Could you check a few things on this model? Use its own coordinates, in mm. A direction names the side the tool comes from. Give positions to 0.01 mm unless a question says otherwise; leave off trailing zeros. Loops run counter-clockwise (first coordinate to the right, second up) from the corner with the lowest first, then second, coordinate; pieces in that order, holes last. Notation, with made-up numbers: (70, 11.25) - (79, 11.25) arc R36 ccw to (79, 45.25) - close; hole circle Ø1 at (26, 47.25). An arc over 180 degrees is marked (long way). Write each question's results on one line, items separated by ' | '. Start each with the question number.
(1) Suppose I cut it at B-B (y = 20). Please give me the cut outline in (x, z).
(2) If we mould it in two halves opening along X, with no side actions, what happens to faces 1 (the face through (-17.7, 43.22, 87.97)), 2 (the face through (52, 43, 117.475)), 3 (the face through (-25.4, 43, 27))? For each: released by +X, released by -X, zero draft, split by the parting line, or undercut.
(3) On a 3-axis mill with a long thin cutter (end or side, diameter ignored), from which of +Z, -Z, +X, -X, +Y, -Y can I reach the whole of each face in a straight line? I mean faces 4 (the face through (0, 20, 3)), 5 (the face through (101.6, 20, 3)), 6 (the face through (50, 20, 6.35)), 7 (the face through (3.175, 43, -39)). Say none if no direction works.
(4) Suppose I cut it at D-D (x = 39). Please give me the cut outline in (y, z) (3 decimals).
(5) Suppose I cut it at C-C (y = 42). Please give me the cut outline in (x, z) (3 decimals), and give its area (3 significant figures).
(6) For pin 1 (20 mm diameter, centred on x = 56.5, y = 18.5, fed in from -Z); pin 2 (2.5 mm diameter, centred on x = 119.2, z = 85.725, fed in from +Y); pin 3 (7 mm diameter, centred on x = 45.5, y = 42, fed in from -Z) (3 decimals); pin 4 (14.5 mm diameter, centred on x = 12.7, y = 20, fed in from +Z), each with a flat end and sliding along its axis, tell me the tip position at first contact or that it passes through.
(7) Suppose I cut it at A-A (x = 88.9). Please give me the cut outline in (y, z) (3 decimals).
(8) I need wall thicknesses on line 1 (X direction, y = 20, z = 1.5); line 2 (Z direction, x = -17.6, y = 44.25) (3 decimals); line 3 (Y direction, x = 64, z = 12.5). Which ranges of each line are inside material? Lowest first, please.
Autodesk Inventor part; units mm, degrees
ref_plane "YZ Plane" through (0, 0, 0) normal (1, 0, 0) x (0, 1, 0)
ref_plane "XZ Plane" through (0, 0, 0) normal (0, 1, 0) x (-1, 0, 0)
ref_plane "XY Plane" through (0, 0, 0) normal (0, 0, 1) x (1, 0, 0)
sketch "Sketch1" plane through (0, 0, 0) normal (0, 0, 1) x (1, 0, 0)
  line L0 (0, 0) -> (101.6, 0)
  line L1 (101.6, 0) -> (101.6, 40)
  line L2 (101.6, 40) -> (0, 40)
  line L3 (0, 40) -> (0, 0)
  dimension "d0" = 101.6
  dimension "d1" = 40
extrude "Mounting Plate" add sketch "Sketch1" along normal blind 6.35
sketch "Sketch2" plane through (0, 40, 0) normal (0, 1, 0) x (1, 0, 0)
  line L0 (0, -6.35) -> (101.6, -6.35)
  line L1 (101.6, 0) -> (101.6, -6.35)
  line L2 (101.6, 0) -> (0, 0)
  line L3 (0, 0) -> (0, -6.35)
  line L4 (-25.4, 66.675) -> (127, 66.675)
  line L5 (127, 66.675) -> (127, -117.475)
  line L6 (127, -117.475) -> (-25.4, -117.475)
  line L7 (-25.4, -117.475) -> (-25.4, 66.675)
  line L8 (3.175, 66.675) -> (98.425, 66.675)
  line L9 (98.425, 66.675) -> (98.425, 12.7)
  line L10 (95.25, 9.525) -> (6.35, 9.525)
  line L11 (3.175, 12.7) -> (3.175, 66.675)
  arc A0 (3.175, 12.7) -> (6.35, 9.525) centre (6.35, 12.7) ccw
  arc A1 (95.25, 9.525) -> (98.425, 12.7) centre (95.25, 12.7) ccw
  point P0 (98.425, 9.525)
  point P1 (3.175, 9.525)
  point P2 (50.8, 66.675)
  point P3 (50.8, 0)
  point P4 (50.8, 9.525)
  dimension "d4" = 152.4
  dimension "d5" = 184.15
  dimension "d6" = 95.25
  dimension "d7" = 57.15
  dimension "d8" = 9.525
  dimension "d9" = 3.175
extrude "Back Plate" add sketch "Sketch2" along normal blind 6.35 contours L3 L2 L1 L0 | L4 L11 A0 L10 A1 L9 L5 L6 L7
sketch "Sketch3" plane through (0, 0, 0) normal (0, 0, -1) x (-1, 0, 0)
  line L0 (0, 0) -> (-101.6, 0)
  line L1 (-101.6, 0) -> (-101.6, 40)
  line L2 (-88.9, 20) -> (-12.7, 20)
  line L3 (-6.35, 40) -> (-95.25, 40)
  point P0 (-50.8, 20)
  point P1 (-50.8, 40)
  dimension "d12" = 76.2
  dimension "d13" = 20
hole "Hole1" at (88.9, 20, 0) at (12.7, 20, 0) direction (0, 0, 1) diameter 8.9916 end through all
sketch "Sketch4" plane through (0, 40, 0) normal (0, -1, 0) x (1, 0, 0)
  line L0 (-25.4, 117.475) -> (127, 117.475)
  line L1 (0, 6.35) -> (101.6, 6.35)
  line L2 (-17.6, 85.725) -> (119.2, 85.725)
  point P0 (50.8, 85.725)
  point P1 (50.8, 117.475)
  dimension "d21" = 136.8
  dimension "d22" = 31.75
hole "Hole2" at (-17.6, 40, 85.725) at (119.2, 40, 85.725) direction (0, 1, 0) diameter 4.4958 end through all
properties part number "LIDAR Bracket"
Output values:
1) outline: (0, 0) - (8.2, 0) - (8.2, 6.35) - (0, 6.35) - close; (17.2, 0) - (84.4, 0) - (84.4, 6.35) - (17.2, 6.35) - close; (93.4, 0) - (101.6, 0) - (101.6, 6.35) - (93.4, 6.35) - close
2) face 1: undercut | face 2: zero draft | face 3: released by -X
3) face 4: +Z, -Z, -X, -Y | face 5: +Z, -Z, +X, -Y | face 6: +Z, +X, -X, -Y | face 7: -Z, +Y, -Y
4) outline: (0, 0) - (40, 0) - (40, -9.525) - (46.35, -9.525) - (46.35, 117.475) - (40, 117.475) - (40, 6.35) - (0, 6.35) - close
5) outline: (-25.4, -66.675) - (3.175, -66.675) - (3.175, -12.7) arc R3.175 cw to (6.35, -9.525) - (95.25, -9.525) arc R3.175 cw to (98.425, -12.7) - (98.425, -66.675) - (127, -66.675) - (127, 117.475) - (-25.4, 117.475) - close; hole circle Ø4.496 at (-17.6, 85.725); hole circle Ø4.496 at (119.2, 85.725) | area: 22,600 mm2
6) pin 1: z = 0 | pin 2: through | pin 3: z = -9.525 | pin 4: z = 6.35
7) outline: (0, 0) - (15.504, 0) - (15.504, 6.35) - (0, 6.35) - close; (24.496, 0) - (40, 0) - (40, -9.525) - (46.35, -9.525) - (46.35, 117.475) - (40, 117.475) - (40, 6.35) - (24.496, 6.35) - close
8) line 1: 0 to 8.2, 17.2 to 84.4, 93.4 to 101.6 | line 2: -66.675 to 83.477, 87.973 to 117.475 | line 3: 40 to 46.35
